The listing builds one solid part. Answer for the finished solid, in the listing's coordinates (mm). A direction names the side the tool comes from. Give positions to 0.01 mm unless a question says otherwise; leave off trailing zeros. Order: outer loops, then holes, each group sorted by start corner. A loop starts at its lowest first (then second) coordinate and runs counter-clockwise, first axis right, second up. Notation, with made-up numbers: (74, 45) - (115, 45) arc R25 ccw to (115, 82) - close; hole circle Ø7 at (9.25, 43.25). An arc over 180 degrees is marked (long way). Use CSV: the item, a comma, the result in double quotes.
Autodesk Inventor part; units mm, degrees
ref_plane "YZ Plane" through (0, 0, 0) normal (1, 0, 0) x (0, 1, 0)
ref_plane "XZ Plane" through (0, 0, 0) normal (0, 1, 0) x (-1, 0, 0)
ref_plane "XY Plane" through (0, 0, 0) normal (0, 0, 1) x (1, 0, 0)
sketch "Sketch1" plane through (0, 0, 0) normal (0, 0, 1) x (1, 0, 0)
  circle A0 centre (0, 0) radius 8.5
  line L0 (-394.9167, 627.0158) -> (-24.6817, -14.25)
  arc A1 (-24.6817, -14.25) -> (24.6817, -14.25) centre (0, 0) ccw
  line L1 (24.6817, -14.25) -> (394.9167, 627.0158)
  arc A2 (394.9167, 627.0158) -> (370.235, 669.7658) centre (370.235, 641.2658) ccw
  line L2 (370.235, 669.7658) -> (-370.235, 669.7658)
  arc A3 (-370.235, 669.7658) -> (-394.9167, 627.0158) centre (-370.235, 641.2658) ccw
  line L3 (0, 0) -> (0, 669.7658) construction
  line L4 (-332.9959, 619.7658) -> (332.9959, 619.7658)
  line L5 (332.9959, 619.7658) -> (0, 43)
  line L6 (0, 43) -> (-332.9959, 619.7658)
  circle A4 centre (-370.235, 641.2658) radius 8.5
  circle A5 centre (370.235, 641.2658) radius 8.5
  dimension "d34" = 17
  dimension "d35" = 20
  dimension "d36" = 740.47
  dimension "d37" = 740.47
  dimension "d38" = 50
extrude "Plate1" add sketch "Sketch1" along normal blind 3
fillet "Corner Round3" radius 6 3 edges at (-332.9959, 619.7658, 1.5) (0, 43, 1.5) (332.9959, 619.7658, 1.5)
equation "\"d37\" = d36"
equation "\"d2\" = Thickness"
equation "\"BendReliefWidth\" = Thickness"
equation "\"BendReliefDepth\" = 0.5 * Thickness"
equation "\"CornerReliefSize\" = 4 * Thickness"
equation "\"MinimumRemnant\" = 2 * Thickness"
equation "\"TransitionRadius\" = BendRadius"
equation "\"JacobiRadiusSize\" = BendRadius"
equation "\"GapSize\" = Thickness"
properties part number "PNS-689 leg floor pattern" material "Stainless Steel"
Item 1: Each of these flat-tipped pins is pushed along its axis until it touches: pin 1 (22 mm diameter, centred on x = 0, y = 0, fed in from -Z); pin 2 (1 mm diameter, centred on y = 236, z = 0.5, fed in from +X). Where does it stop, or does it pass through?
Taken from the geometry:
pin 1,"z = 0"
pin 2,"x = 169.45"
Item 2: The part is cut by section A-A (x = -245.5). Give the vertices of the cut face in (y, z).
Taken from the geometry:
outline,"(368.22, 0) - (468.22, 0) - (468.22, 3) - (368.22, 3) - close; (619.77, 0) - (669.77, 0) - (669.77, 3) - (619.77, 3) - close"
Item 3: The part is cut by section B-B (y = 304). Give the vertices of the cut face in (x, z).
Taken from the geometry:
outline,"(-208.42, 0) - (-150.69, 0) - (-150.69, 3) - (-208.42, 3) - close; (150.69, 0) - (208.42, 0) - (208.42, 3) - (150.69, 3) - close"
Item 4: The part is cut by section C-C (z = 1.2). Give the vertices of the cut face in (x, y) (3 decimals), and give its area (3 significant figures).
Taken from the geometry:
outline,"(-394.917, 627.016) - (-24.682, -14.25) arc R28.5 ccw to (24.682, -14.25) - (394.917, 627.016) arc R28.5 ccw to (370.235, 669.766) - (-370.235, 669.766) arc R28.5 ccw to start; hole circle Ø17 at (-370.235, 641.266); hole (-327.8, 610.766) - (-5.196, 52) arc R6 ccw to (5.196, 52) - (327.8, 610.766) arc R6 ccw to (322.604, 619.766) - (-322.604, 619.766) arc R6 ccw to start; hole circle Ø17 at (0, 0); hole circle Ø17 at (370.235, 641.266)"
area,"111,000 mm^2"
Item 5: Find the intervals of material crossed by line 1 along Y through (x, z) = (107, 2.5); line 2 along Y through (x, z) = (-277.5, 2.75); line 3 along X through (y, z) = (549, 1.9), in increasing order.
Taken from the geometry:
line 1,"128.33 to 228.33, 619.77 to 669.77"
line 2,"423.64 to 523.64, 619.77 to 669.77"
line 3,"-349.87 to -292.14, 292.14 to 349.87"
Item 6: The mould has two halves that part along Y. Classify faces 3 (the face through (-395.123, 655.152, 1.479)), 4 (the face through (-150, 296, 0)), 5 (the face through (-366.3, 648.8, 1.5)), 6 (the face through (-164.24, 327.47, 1.48)): +Y half, -Y half, draft (parallel to the pull), parting line (faces both ways), or undercut.
Taken from the geometry:
face 3,"parting line"
face 4,"draft"
face 5,"undercut"
face 6,"undercut"
Item 7: Which of the six approach directions +Z, -Z, +X, -X, +Y, -Y give full straight-line access (tool end or side, diameter ignored) to faces 1 (the face through (168.756, 335.294, 1.479)), 2 (the face through (207.208, 301.894, 1.479))?
Taken from the geometry:
face 1,"+Z, -Z"
face 2,"+Z, -Z, +X, -Y"
